Geometry: final body of the model. Coordinates: model frame, mm. Face numbers are marked on the shaded views. Round coordinates to 2 decimals unless told otherwise and drop trailing zeros. Write each loop counter-clockwise with the first axis right and the second up, starting at its lowest first coordinate (ties: lowest second). Pieces come first, ordered by that corner, then holes. Notation, with made-up numbers: M 79.5,84 L 98.5,84 A20 ccw 98.5,106 Z; hole C -2.75,15 d5. An arc over 180 degrees is marked long. Use one line per item in the form item = value. Start each with the question number.
Item 1: Pin query (flat end, axial travel): pin 1 Ø1 at (x, z) = (2, -7) entering from +Y; pin 2 Ø1.5 at (y, z) = (8.5, 4.5) entering from -X; pin 3 Ø1.5 at (y, z) = (8, -0.5) entering from -X. Return the tip coordinate at first contact, or that it passes through.
Item 2: Pull-direction query (X, two-part tool) for the marked faces 1, 2 and 3; classes: pulls with the +X half, pulls with the -X half, needs draft (parallel to the pull), parting line crosses it, or undercut.
Item 3: Section query A-A (z = 2.25). Return loops of the section in (x, y).
Item 4: Section query C-C (y = 11.75). Return loops of the section in (x, z), and give its area (3 significant figures).
Item 5: Section query D-D (z = -4.5). Return loops of the section in (x, y), and give its area (3 significant figures).
Item 6: Ray query, probe 1 along Z at (x, y) = (0, 5.65); probe 2 along Z at (x, y) = (0, 11.25); probe 3 along Y at (x, z) = (10.25, 2.5). Return the intervals inside material, ascending.
Item 7: Section query B-B (x = 0). Return loops of the section in (y, z), and give its area (3 significant figures).
from build123d import *

# Parameters (mm, degrees)
SKETCH1_R           = 6.2
SKETCH1_R_2         = 5.2
BOSS_EXTRUDE1_DEPTH = 14
SKETCH2_R           = 12
SKETCH2_R_2         = 1.25
SKETCH2_R_3         = 5.2
BOSS_EXTRUDE2_DEPTH = 1.25


with BuildPart() as part:
    # Sketch1 → Boss-Extrude1 (new body)
    with BuildSketch(Plane(origin=(0, 0, 0), x_dir=(1, 0, 0), z_dir=(0, 1, 0))):
        Circle(SKETCH1_R)
        Circle(SKETCH1_R_2, mode=Mode.SUBTRACT)
    extrude(amount=BOSS_EXTRUDE1_DEPTH)

    # Sketch2 → Boss-Extrude2 (add)
    with BuildSketch(Plane(origin=(0, 4.999999906, 0), x_dir=(-1, 0, 0), z_dir=(0, 1, 0))):
        Circle(SKETCH2_R)
        with Locations((0, -9)):
            Circle(SKETCH2_R_2, mode=Mode.SUBTRACT)
        with Locations((-7.794228634, 4.5)):
            Circle(SKETCH2_R_2, mode=Mode.SUBTRACT)
        with Locations((7.794228634, 4.5)):
            Circle(SKETCH2_R_2, mode=Mode.SUBTRACT)
        Circle(SKETCH2_R_3, mode=Mode.SUBTRACT)
    extrude(amount=BOSS_EXTRUDE2_DEPTH)


solid = part.part
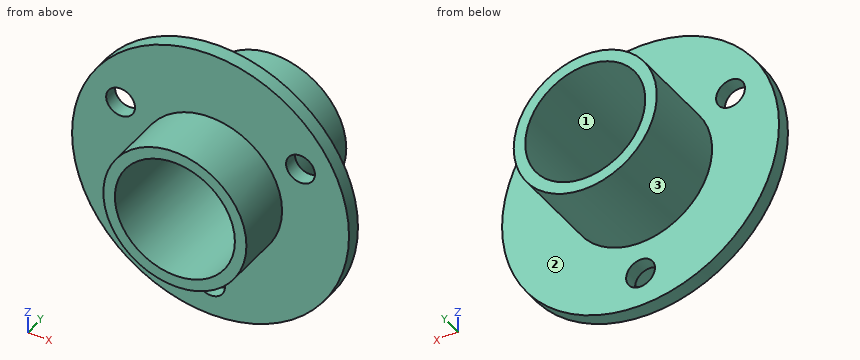
Working result:
q1.pin_1 = 6.25
q1.pin_2 = -4.94
q1.pin_3 = -6.2
q2.face_1 = undercut
q2.face_2 = needs draft
q2.face_3 = parting line crosses it
q3.outline = M -11.79,5 L -5.78,5 L -5.78,0 L -4.69,0 L -4.69,14 L -5.78,14 L -5.78,6.25 L -11.79,6.25 Z; M 4.69,0 L 5.78,0 L 5.78,5 L 11.79,5 L 11.79,6.25 L 5.78,6.25 L 5.78,14 L 4.69,14 Z
q4.outline = C 0,0 d12.4; hole C 0,0 d10.4
q4.area = 35.8 mm²
q5.outline = M -11.12,5 L -4.26,5 L -4.26,0 L -2.61,0 L -2.61,14 L -4.26,14 L -4.26,6.25 L -11.12,6.25 Z; M 2.61,0 L 4.26,0 L 4.26,5 L 11.12,5 L 11.12,6.25 L 4.26,6.25 L 4.26,14 L 2.61,14 Z
q5.area = 63.6 mm²
q6.probe_1 = -12 to -10.25, -7.75 to -5.2, 5.2 to 12
q6.probe_2 = -6.2 to -5.2, 5.2 to 6.2
q6.probe_3 = 5 to 6.25
q7.outline = M 0,-6.2 L 5,-6.2 L 5,-7.75 L 6.25,-7.75 L 6.25,-6.2 L 14,-6.2 L 14,-5.2 L 0,-5.2 Z; M 0,5.2 L 14,5.2 L 14,6.2 L 6.25,6.2 L 6.25,12 L 5,12 L 5,6.2 L 0,6.2 Z; M 5,-12 L 6.25,-12 L 6.25,-10.25 L 5,-10.25 Z
q7.area = 39.4 mm²
